from build123d import *

# Parameters (mm, degrees)
F1_DEPTH      = 228.6
F2_W          = 12.7
F2_H          = 6.35
F3_DEPTH      = 11.938
F3_DEPTH_BACK = 25.4
F4_R          = 2.579688
F5_DEPTH      = 12.7


with BuildPart() as f1:
    # F0 (on Front) → F1 (new body)
    with BuildSketch(Plane.XZ):
        with BuildLine():
            ThreePointArc((10.071912, -2.38125), (9.37446, -0.697452), (7.690662, 0))
            Line((7.690662, 0), (-0.246838, 0))
            ThreePointArc((-0.246838, 0), (-1.930636, -0.697452), (-2.628088, -2.38125))
            Line((-2.628088, -2.38125), (-2.628088, -10.31875))
            ThreePointArc((-2.628088, -10.31875), (-1.930636, -12.002548), (-0.246838, -12.7))
            Line((-0.246838, -12.7), (7.690662, -12.7))
            ThreePointArc((7.690662, -12.7), (9.37446, -12.002548), (10.071912, -10.31875))
            Line((10.071912, -10.31875), (10.071912, -2.38125))
        make_face()
        with BuildLine():
            Line((0.546912, -1.5875), (6.896912, -1.5875))
            ThreePointArc((6.896912, -1.5875), (8.019444, -2.052468), (8.484412, -3.175))
            Line((8.484412, -3.175), (8.484412, -9.525))
            ThreePointArc((8.484412, -9.525), (8.019444, -10.647532), (6.896912, -11.1125))
            Line((6.896912, -11.1125), (0.546912, -11.1125))
            ThreePointArc((0.546912, -11.1125), (-0.57562, -10.647532), (-1.040588, -9.525))
            Line((-1.040588, -9.525), (-1.040588, -3.175))
            ThreePointArc((-1.040588, -3.175), (-0.57562, -2.052468), (0.546912, -1.5875))
        make_face(mode=Mode.SUBTRACT)
    extrude(amount=F1_DEPTH)

    # F2 (on Right) → F3 (cut, two sides)
    with BuildSketch(Plane.YZ) as f3_sk:
        with Locations((-215.9, -3.175)):
            Rectangle(F2_W, F2_H)
        with Locations((-12.7, -3.175)):
            Rectangle(F2_W, F2_H)
    extrude(amount=F3_DEPTH, mode=Mode.SUBTRACT)
    extrude(f3_sk.sketch, amount=-F3_DEPTH_BACK, mode=Mode.SUBTRACT)

    # F4 (on Top) → F5 (cut)
    with BuildSketch(Plane.XY):
        with Locations((3.721912, -12.7)):
            Circle(F4_R)
        with Locations((3.721912, -215.9)):
            Circle(F4_R)
    extrude(amount=-F5_DEPTH, mode=Mode.SUBTRACT)


solid = f1.part
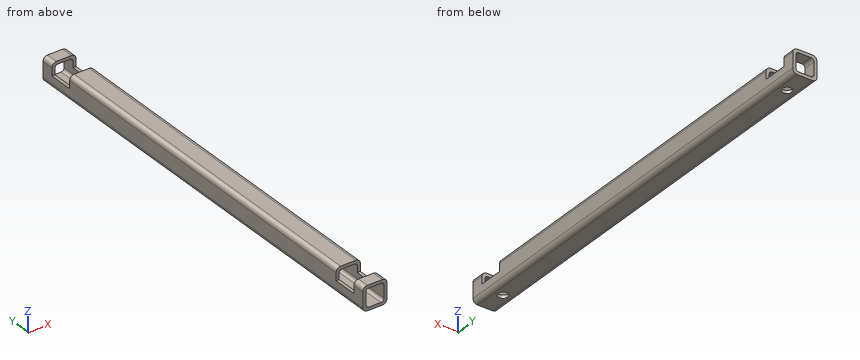
Verification items for the finished model (mm, model axes). Coordinates: 2 decimals unless noted, no trailing zeros. Write each loop counter-clockwise with the first axis right and the second up, starting at its lowest first coordinate (ties: lowest second). Pieces come first, ordered by that corner, then holes. Notation, with made-up numbers: (66, 8) -> (102, 8) arc R13 cw to (102, 23) -> close; hole circle Ø9 at (78, 2). An arc over 180 degrees is marked (long way). One line per item, written item: value. Start each with the question number.
Q1. Cross-section at B-B on y = -56. Enter the section's corners in (x, z) (1 decimal), and give its area (3 significant figures).
Q2. Go/stop test with flat-tipped pins: P1, Ø1, axis at x = 2, y = -192.5, coming from the +Z side; P2, Ø0.8, axis at x = 9.5, y = -10, coming from the +Z side; P3, Ø6.5, axis at x = 3.72, y = -215.9, coming from the +Z side; P4, Ø1, axis at y = -199.5, z = -1.5, coming from the -X side. Record where each tip stops, or that it passes through.
Q3. Thickness scan on L1, parallel to Y at x = 9, z = -3.75; L2, parallel to X at y = -198.5, z = -6; L3, parallel to Z at x = 4.75, y = -30.5. Record the ranges inside material, lowest first. Write a range as from..to.
Checked values:
1. outline: (-2.6, -10.3) arc R2.4 ccw to (-0.2, -12.7) -> (7.7, -12.7) arc R2.4 ccw to (10.1, -10.3) -> (10.1, -2.4) arc R2.4 ccw to (7.7, 0) -> (-0.2, 0) arc R2.4 ccw to (-2.6, -2.4) -> close; hole (-1, -9.5) arc R1.6 ccw to (0.5, -11.1) -> (6.9, -11.1) arc R1.6 ccw to (8.5, -9.5) -> (8.5, -3.2) arc R1.6 ccw to (6.9, -1.6) -> (0.5, -1.6) arc R1.6 ccw to (-1, -3.2) -> close
1. area: 67.9 mm²
2. P1: stops at z = 0
2. P2: stops at z = -6.35
2. P3: stops at z = -11.11
2. P4: stops at x = -2.6
3. L1: y = -228.6..-222.25, -209.55..-19.05, -6.35..0
3. L2: x = -2.63..-1.04, 8.48..10.07
3. L3: z = -12.7..-11.11, -1.59..0
